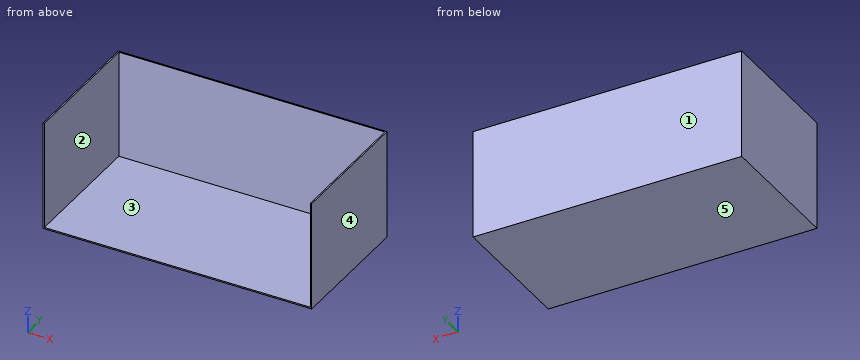
from build123d import *

# Parameters (mm, degrees)
F0_W     = 508
F0_H     = 254
F1_DEPTH = 2.54
F2_W     = 2.54
F2_H     = 254
F3_DEPTH = 203.2
F5_DEPTH = 203.2
F6_W     = 2.54
F6_H     = 251.46
F7_DEPTH = 203.2


with BuildPart() as f1:
    # F0 (on Top) → F1 (new body)
    with BuildSketch(Plane.XY):
        Rectangle(F0_W, F0_H)
    extrude(amount=F1_DEPTH)

    # F2 (on face) → F3 (join)
    with BuildSketch(Plane.XY.offset(2.54)):
        with Locations((-252.73, 0)):
            Rectangle(F2_W, F2_H)
    extrude(amount=F3_DEPTH)

    # F4 (on face) → F5 (join)
    with BuildSketch(Plane.XY.offset(2.54)):
        Polygon((254, 124.46), (254, 127), (-49.611485, 127), (-251.46, 127), (-251.46, 124.46), align=None)
    extrude(amount=F5_DEPTH)

    # F6 (on face) → F7 (join)
    with BuildSketch(Plane.XY.offset(2.54)):
        with Locations((252.73, -1.27)):
            Rectangle(F6_W, F6_H)
    extrude(amount=F7_DEPTH)


solid = f1.part
Verification items for the finished model (mm, model axes). Face numbers are marked on the shaded views. A direction names the side the tool comes from. Coordinates: 2 decimals unless noted, no trailing zeros. Order: outer loops, then holes, each group sorted by start corner. A loop starts at its lowest first (then second) coordinate and runs counter-clockwise, first axis right, second up. Notation, with made-up numbers: M 32.5,64 L 68.5,64 A22 ccw 68.5,97 Z; hole C 48,-19.5 d3. An arc over 180 degrees is marked long. One line per item, written item: value. Start each with the question number.
Item 1: Thickness scan on probe 1 along X at (y, z) = (60.5, 82); probe 2 along Z at (x, y) = (213.5, 100); probe 3 along Y at (x, z) = (-159.5, 12). Record the ranges inside material, lowest first.
Item 2: Sectioned sample at C-C on x = -32. Record the cut outline in (y, z).
Item 3: Sectioned sample at B-B on z = 72. Record the cut outline in (x, y), then the cut area to 3 significant figures.
Item 4: Sectioned sample at A-A on y = 27. Record the cut outline in (x, z), then the cut area to 3 significant figures.
Item 5: Depth check by flat-ended pin: P1, Ø8, axis at x = 45, z = 35, coming from the -Y side. Enter the tip coordinate at first touch or a pass-through.
Item 6: Mould release check, pull along X, two halves, no side actions. Record for the marked faces 3, 4 and 5: pulls with the +X half, pulls with the -X half, needs draft (parallel to the pull), parting line crosses it, or undercut.
Item 7: Access from +Z, -Z, +X, -X, +Y, -Y to the whole of each face (thin tool, end or side, straight path). Record for the marked faces 1 and 2.
Calculated:
1. probe 1: -254 to -251.46, 251.46 to 254
1. probe 2: 0 to 2.54
1. probe 3: 124.46 to 127
2. outline: M -127,0 L 127,0 L 127,205.74 L 124.46,205.74 L 124.46,2.54 L -127,2.54 Z
3. outline: M -254,-127 L -251.46,-127 L -251.46,124.46 L 251.46,124.46 L 251.46,-127 L 254,-127 L 254,127 L -254,127 Z
3. area: 2,570 mm^2
4. outline: M -254,0 L 254,0 L 254,205.74 L 251.46,205.74 L 251.46,2.54 L -251.46,2.54 L -251.46,205.74 L -254,205.74 Z
4. area: 2,320 mm^2
5. P1: y = 124.46
6. face 3: undercut
6. face 4: pulls with the +X half
6. face 5: needs draft
7. face 1: +Z, -Z, +X, -X, +Y
7. face 2: +Z, -Y
